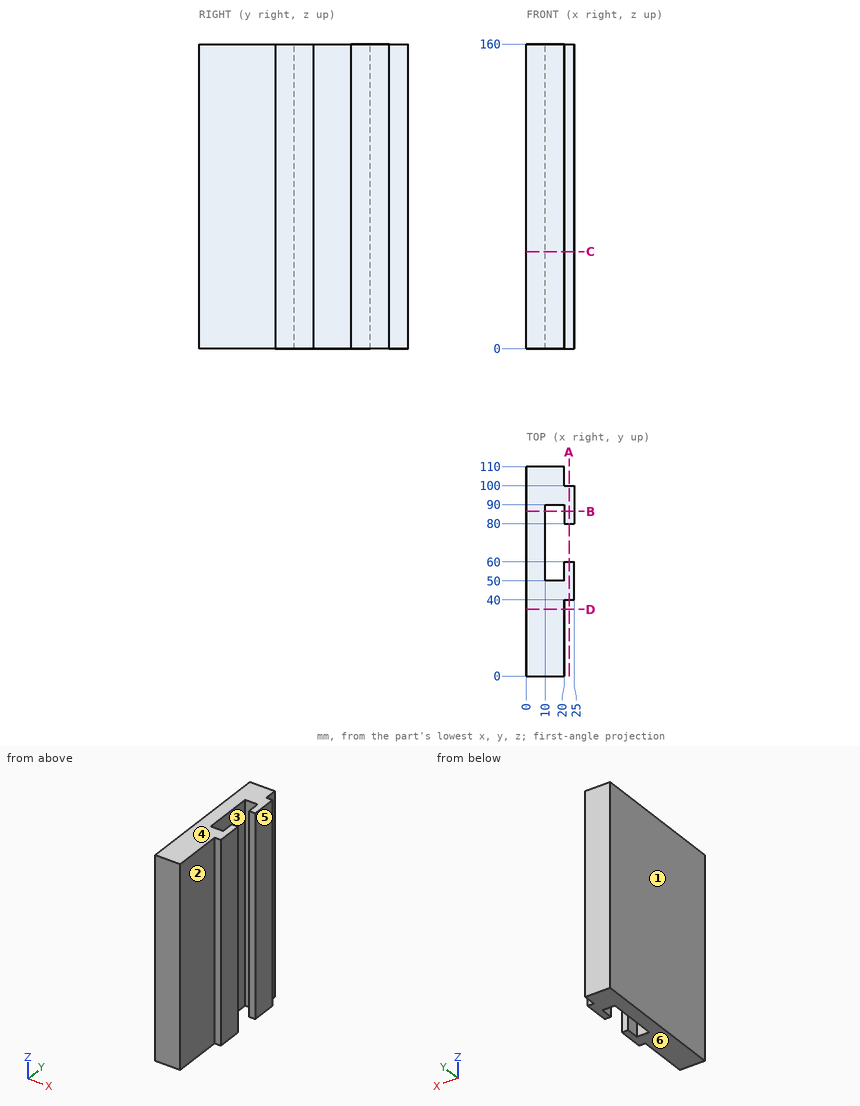
Drawing for the job (mm, zero at the part's lowest x, y, z). A direction names the side the tool comes from. Coordinates: 2 decimals unless noted, no trailing zeros. Write each loop counter-clockwise with the first axis right and the second up, starting at its lowest first coordinate (ties: lowest second). Pieces come first, ordered by that corner, then holes. Notation, with made-up numbers: (-18, 71.5) -> (23, 71.5) arc R33 cw to (23, 100.5) -> close; hole circle Ø2 at (-6, 11). An arc over 180 degrees is marked (long way). One line per item, written item: value. Start each with the question number.
1) Slice it at A-A on x = 22.5. Write the cut outline in (y, z), then the cut area to 3 significant figures.
2) Pull direction Z, two halves, no side cores. Call the marked faces 4, 5 and 6: +Z half, -Z half, draft (parallel to the pull), parting line (faces both ways), or undercut.
3) Which spindle directions (+Z, -Z, +X, -X, +Y, -Y) get a long thin tool onto all of the face, cutting with end or side? Do the marked faces 1, 2 and 3. Say none if no direction does.
4) Slice it at C-C on z = 51. Write the cut outline in (x, y), then the cut area to 3 significant figures.
5) Slice it at D-D on y = 35. Write the cut outline in (x, z), then the cut area to 3 significant figures.
6) Probe probe 1 along Y at (x, z) = (20.5, 91.5); probe 2 along X at (y, z) = (58, 32); probe 3 along Y at (x, z) = (11.5, 36). List the from-to ranges inside material, lowest first.
7) Flat gauge pins, fed straight in: pin 1 Ø4 at (x, z) = (22.5, 68.5) entering from -Y; pin 2 Ø3 at (y, z) = (107, 66) entering from +X; pin 3 Ø1.5 at (x, z) = (22.5, 54) entering from +Y. Where does each tip first touch, or does it go through?
8) Slice it at B-B on y = 86.5. Write the cut outline in (x, z), then the cut area to 3 significant figures.
Answers follow:
1. outline: (40, 0) -> (60, 0) -> (60, 160) -> (40, 160) -> close; (80, 0) -> (100, 0) -> (100, 160) -> (80, 160) -> close
1. area: 6,400 mm2
2. face 4: +Z half
2. face 5: draft
2. face 6: -Z half
3. face 1: +Z, -Z, -X, +Y, -Y
3. face 2: +Z, -Z, +X, -Y
3. face 3: +Z, -Z
4. outline: (0, 0) -> (20, 0) -> (20, 40) -> (25, 40) -> (25, 60) -> (20, 60) -> (20, 50) -> (10, 50) -> (10, 90) -> (20, 90) -> (20, 80) -> (25, 80) -> (25, 100) -> (20, 100) -> (20, 110) -> (0, 110) -> close
4. area: 2,000 mm2
5. outline: (0, 0) -> (20, 0) -> (20, 160) -> (0, 160) -> close
5. area: 3,200 mm2
6. probe 1: 40 to 60, 80 to 100
6. probe 2: 0 to 10, 20 to 25
6. probe 3: 0 to 50, 90 to 110
7. pin 1: y = 40
7. pin 2: x = 20
7. pin 3: y = 100
8. outline: (0, 0) -> (10, 0) -> (10, 160) -> (0, 160) -> close; (20, 0) -> (25, 0) -> (25, 160) -> (20, 160) -> close
8. area: 2,400 mm2
